from build123d import *

# Parameters (mm, degrees)
SZKIC2_R                   = 1
WYTNIJ_WYCI_GNI_CIE1_DEPTH = 10


with BuildPart() as part:
    # Szkic1 → Obrót1 (revolve)
    with BuildSketch(Plane.XY):
        Polygon((-10.055, -7), (-10.055, 0), (-75, 0), (-75, -6), (-59.4, -6), (-59.4, -2.9), (-54, -2.9), (-54, -6), (-50, -6), (-50, -7.2), (-46.9, -7.2), (-46.9, -12.5), (-50, -12.5), (-50, -14.251552945), (-45, -14.251552945), (-43.721355564, -7), align=None)
    revolve(axis=Axis((0, 0, 0), (0, -1, 0)))

    # Szkic2 → Wytnij-wyciągnięcie1 (cut)
    with BuildSketch(Plane.XZ.offset(6)):
        with Locations((0.44346391, 51.984815166)):
            Circle(SZKIC2_R)
    extrude(amount=-WYTNIJ_WYCI_GNI_CIE1_DEPTH, mode=Mode.SUBTRACT)


solid = part.part
Can you work these out from the model? Positions are in its coordinate system, mm. A direction names the side the tool comes from. Give positions to 0.01 mm unless a question says otherwise; leave off trailing zeros. Order: outer loops, then holes, each group sorted by start corner. A loop starts at its lowest first (then second) coordinate and runs counter-clockwise, first axis right, second up. Notation, with made-up numbers: M -17.5,39 L -12.5,39 A20 cw -12.5,75 Z; hole C 30.25,53 d6. An arc over 180 degrees is marked long. Use one line per item in the form item = value.
Item 1: Thinking about a two-plate mould opening in Y: for faces 1 (the cylindrical face through (9.764, -3.042, -74.362)), 2 (the flat face through (23, -6, -56)), 3 (the flat face through (45, -7.2, 15)), which applies, pulls with the +Y half, pulls with the -Y half, needs draft (parallel to the pull), parting line crosses it, or undercut?
Values follow:
face_1 = needs draft
face_2 = pulls with the -Y half
face_3 = undercut
Item 2: Will these pins go through, and if not, where does the flat tip stop? pin 1 Ø2 at (x, y) = (26.5, -6) entering from +Z; pin 2 Ø5 at (x, y) = (-34, -11.5) entering from -Z; pin 3 Ø12 at (x, z) = (53, -47.5) entering from -Y; pin 4 Ø12 at (x, z) = (0, 0) entering from -Y.
Values follow:
pin_1 = 70.53
pin_2 = -38.66
pin_3 = -6
pin_4 = through
Item 3: If we section it at B-B, the plane z = 65.5: Write out the boundary of the cut face in (x, y).
Values follow:
outline = M -36.53,-6 L 36.53,-6 L 36.53,0 L -36.53,0 Z
Item 4: If I drill on line 1 along X through (y, z) = (-3.95, 0) (3 decimals); line 2 along X through (y, z) = (-2, 0) (3 decimals); line 3 along Y through (x, z) = (-30, 38), over which ranges is the centre line in solid material (lowest first)? Write a range as [from, to].
Values follow:
line_1 = [-75, -59.4], [-54, -10.055], [10.055, 54], [59.4, 75]
line_2 = [-75, -10.055], [10.055, 75]
line_3 = [-14.25, -12.5], [-7.2, 0]
Item 5: For faces 4 (the flat face through (41, -14.252, -19)), 5 (the cylindrical face through (-47.69, -13.39, -15.02)), 6 (the cylindrical face through (-44.734, -9.887, -14.087)), which set-ups out of +Z, -Z, +X, -X, +Y, -Y let a thin tool reach every point of the face, with its end or its side?
Values follow:
face_4 = +Z, -Z, +X, -X, -Y
face_5 = -Y
face_6 = none
